Here's how the part is built. I have some questions about the finished solid (model axes, mm). A direction names the side the tool comes from. Round coordinates to 2 decimals unless told otherwise and drop trailing zeros. Order: outer loops, then holes, each group sorted by start corner. A loop starts at its lowest first (then second) coordinate and runs counter-clockwise, first axis right, second up.
```python
from build123d import *

# Parameters (mm, degrees)
CUT_EXTRUDE1_DEPTH      = 83.029585714
CUT_EXTRUDE1_DEPTH_BACK = 83.029585714
SKETCH2_R               = 3.175


with BuildPart() as part:
    # Sketch1 → Revolve1 (revolve)
    with BuildSketch(Plane(origin=(0, 0, 0), x_dir=(1, 0, 0), z_dir=(0, 1, 0))):
        Polygon((0, 81.270247818), (-7.874, 81.270247818), (-7.874, 65.522247818), (-4.7625, 65.522247818), (-4.7625, -55.127752182), (-3.175, -55.127752182), (-3.175, -66.303752182), (-1.27, -66.303752182), (-1.27, -57.942062416), (0, -57.942062416), align=None)
    revolve(axis=Axis((0, 0, -59.310994764), (0, 0, 1)))

    # Sketch2 → Cut-Extrude1 (cut, two sides: drawn at the far end of the back side and taken through both)
    with BuildSketch(Plane(origin=(0, 0, 0), x_dir=(1, 0, 0), z_dir=(0, 1, 0)).offset(-CUT_EXTRUDE1_DEPTH_BACK)):
        with Locations(Location((0, 73.396247818, 0), (0, 0, 270))):
            Circle(SKETCH2_R)
    extrude(amount=CUT_EXTRUDE1_DEPTH + CUT_EXTRUDE1_DEPTH_BACK, mode=Mode.SUBTRACT)


solid = part.part
```
1. If we section it at C-C, the plane z = -50: Write out the boundary of the cut face in (x, y) (1 decimal).
Evaluation:
outline: circle Ø9.5 at (0, 0)
2. If we section it at A-A, the plane x = 0: Write out the boundary of the cut face in (y, z) (1 decimal), and give its area (3 significant figures).
Evaluation:
outline: (-7.9, -81.3) - (7.9, -81.3) - (7.9, -76.6) - (-7.9, -76.6) - close; (-7.9, -70.2) - (7.9, -70.2) - (7.9, -65.5) - (4.8, -65.5) - (4.8, 55.1) - (3.2, 55.1) - (3.2, 66.3) - (1.3, 66.3) - (1.3, 57.9) - (-1.3, 57.9) - (-1.3, 66.3) - (-3.2, 66.3) - (-3.2, 55.1) - (-4.8, 55.1) - (-4.8, -65.5) - (-7.9, -65.5) - close
area: 1,350 mm2
3. If we mould it in two halves opening along Y, with no side actions, what happens to faces 3 (the flat face through (0, 0, 57.942)), 4 (the flat face through (0, 5, -65.522)), 5 (the cylindrical face through (-7.27, 3.02, -73.29)), 6 (the cylindrical face through (0.17, -1.26, 62.06))? For each: released by +Y, released by -Y, zero draft, split by the parting line, or undercut.
Evaluation:
face 3: undercut
face 4: zero draft
face 5: split by the parting line
face 6: undercut
4. I'm going to push flat-ended pins straight in: P1, Ø4, axis at x = -1.5, z = -1.5, coming from the +Y side; P2, Ø5, axis at y = 1, z = -56, coming from the -X side; P3, Ø6, axis at y = -4, z = 41.5, coming from the +X side. Where does each tip first touch, or does it pass through?
Evaluation:
P1: stops at y = 4.76
P2: stops at x = -4.76
P3: stops at x = 4.66
5. I need wall thicknesses on probe 1 along Z at (x, y) = (0, 3.5); probe 2 along Z at (x, y) = (0, 3); probe 3 along X at (y, z) = (0, 60.25) (3 decimals). Which ranges of each line are inside material? Lowest first, please.
Evaluation:
probe 1: z = -81.27 to -76.57, -70.22 to 55.13
probe 2: z = -81.27 to -76.57, -70.22 to 66.3
probe 3: x = -3.175 to -1.27, 1.27 to 3.175
6. If we section it at D-D, the plane x = 6.25: Write out the boundary of the cut face in (y, z), and give its area (3 significant figures).
Evaluation:
outline: (-4.79, -81.27) - (4.79, -81.27) - (4.79, -65.52) - (-4.79, -65.52) - close
area: 151 mm2
7. On a 3-axis mill with a long thin cutter (end or side, diameter ignored), from which of +Z, -Z, +X, -X, +Y, -Y can I reach the whole of each face in a straight line? I mean faces 1 (the flat face through (0, 0, -81.27)), 2 (the cylindrical face through (3.78, 2.9, -4.35)). Say none if no direction works.
Evaluation:
face 1: -Z, +X, -X, +Y, -Y
face 2: +Z
